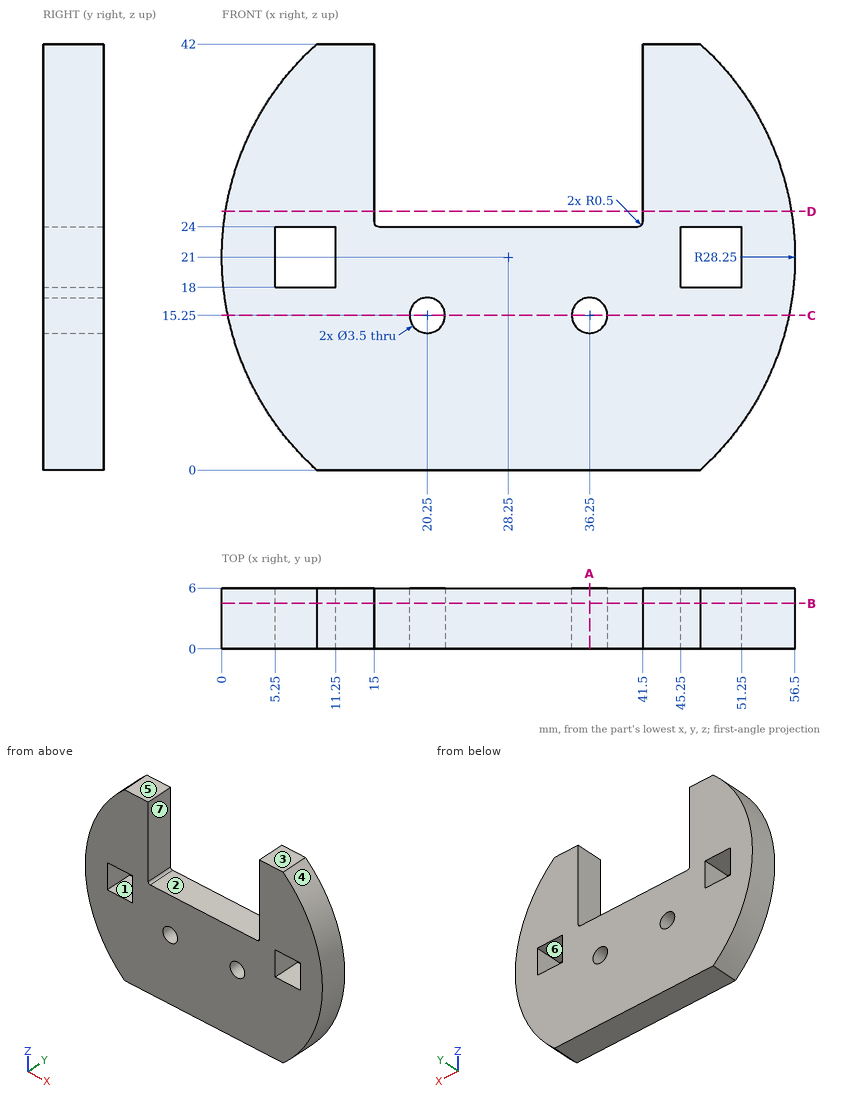
Can you work these out from the drawing? Everything is in mm from the part's minimum corner. A direction names the side the tool comes from. Coordinates: 2 decimals unless noted, no trailing zeros. Write each loop counter-clockwise with the first axis right and the second up, starting at its lowest first coordinate (ties: lowest second). Pieces come first, ordered by that corner, then holes. Notation, with made-up numbers: (55, 52.5) -> (87, 52.5) arc R21 cw to (87, 70.5) -> close; hole circle Ø10 at (79.25, 55.5). An arc over 180 degrees is marked (long way). Write item = value, one per line.
(1) Imagine slicing it at B-B (y = 4.5). Please give me the cut outline in (x, z), and give its area (3 significant figures).
Verdict:
outline = (9.35, 0) -> (47.15, 0) arc R28.25 ccw to (47.15, 42) -> (41.5, 42) -> (41.5, 24.5) arc R0.5 cw to (41, 24) -> (15.5, 24) arc R0.5 cw to (15, 24.5) -> (15, 42) -> (9.35, 42) arc R28.25 ccw to start; hole (5.25, 18) -> (11.25, 18) -> (11.25, 24) -> (5.25, 24) -> close; hole circle Ø3.5 at (20.25, 15.25); hole circle Ø3.5 at (36.25, 15.25); hole (45.25, 18) -> (51.25, 18) -> (51.25, 24) -> (45.25, 24) -> close
area = 1,560 mm^2
(2) On a 3-axis mill with a long thin cutter (end or side, diameter ignored), from which of +Z, -Z, +X, -X, +Y, -Y can I reach the whole of each face in a straight line? I mean the marked faces 5, 6 and 7. Say none if no direction works.
Verdict:
face_5 = +Z, +X, -X, +Y, -Y
face_6 = +Y, -Y
face_7 = +Z, +Y, -Y
(3) Imagine slicing it at A-A (x = 36.25). Please give me the cut outline in (y, z).
Verdict:
outline = (0, 0) -> (6, 0) -> (6, 13.5) -> (0, 13.5) -> close; (0, 17) -> (6, 17) -> (6, 24) -> (0, 24) -> close
(4) Thinking about a two-plate mould opening in X: for the marked faces 1, 2, 3 and 4, which applies, +X half, -X half, draft (parallel to the pull), parting line (faces both ways), or undercut?
Verdict:
face_1 = undercut
face_2 = undercut
face_3 = draft
face_4 = +X half
(5) For pin 1 (1 mm diameter, centred on y = 3.5, z = 22.5, fed in from -X); pin 2 (3 mm diameter, centred on y = 4, z = 37.5, fed in from -X); pin 3 (2 mm diameter, centred on y = 3.5, z = 19, fed in from +X), each with a flat end and sliding along its axis, tell me the tip position at first contact or that it passes through.
Verdict:
pin_1 = 0.02
pin_2 = 4.31
pin_3 = 56.48
(6) If I drill on probe 1 along X at (y, z) = (3.8, 21.5); probe 2 along X at (y, z) = (5.4, 16); probe 3 along Z at (x, y) = (46, 1.7), over which ranges is the centre line in solid material (lowest first)?
Verdict:
probe_1 = 0 to 5.25, 11.25 to 45.25, 51.25 to 56.5
probe_2 = 0.45 to 18.67, 21.83 to 34.67, 37.83 to 56.05
probe_3 = 0 to 18, 24 to 42
(7) Imagine slicing it at C-C (z = 15.25). Please give me the cut outline in (x, y), and give its area (3 significant figures).
Verdict:
outline = (0.59, 0) -> (18.5, 0) -> (18.5, 6) -> (0.59, 6) -> close; (22, 0) -> (34.5, 0) -> (34.5, 6) -> (22, 6) -> close; (38, 0) -> (55.91, 0) -> (55.91, 6) -> (38, 6) -> close
area = 290 mm^2
(8) Imagine slicing it at D-D (z = 25.5). Please give me the cut outline in (x, y).
Verdict:
outline = (0.36, 0) -> (15, 0) -> (15, 6) -> (0.36, 6) -> close; (41.5, 0) -> (56.14, 0) -> (56.14, 6) -> (41.5, 6) -> close
